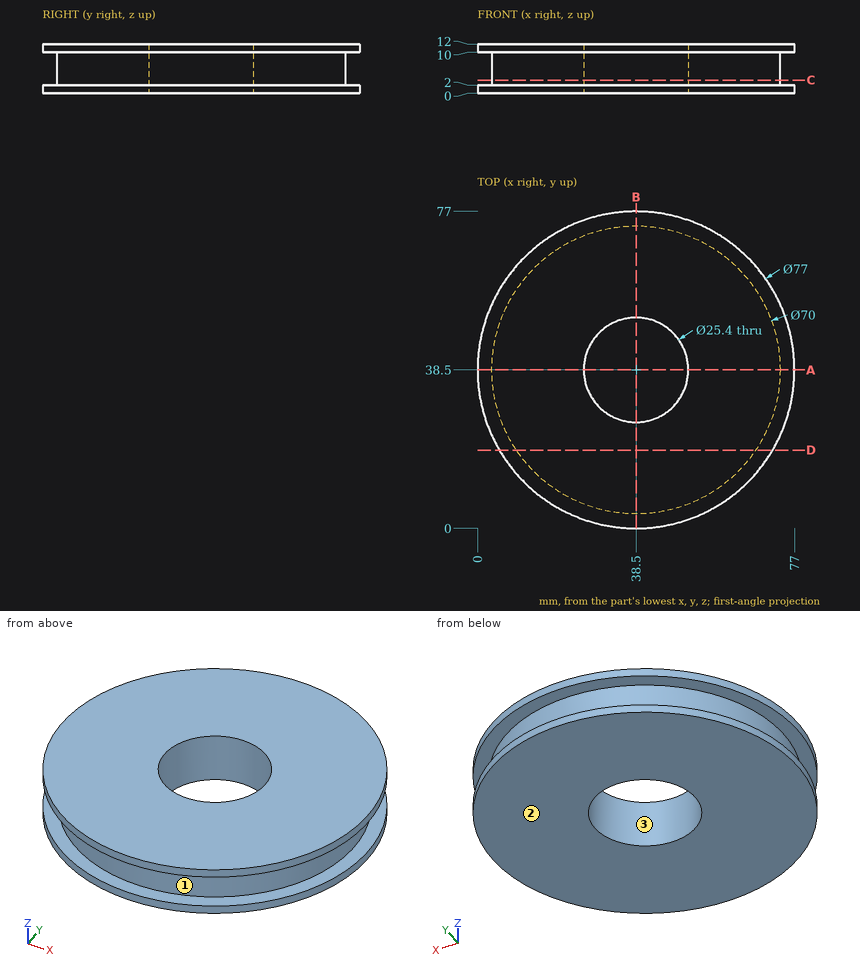
Geometry check sheet. Reference: drawing and pictorial views, mm from the part's lowest x, y, z. Round coordinates to 2 decimals unless told otherwise and drop trailing zeros. Loops run counter-clockwise (first coordinate to the right, second up) from the corner with the lowest first, then second, coordinate; pieces in that order, holes last. Notation, with made-up numbers: M -15,64 L 28,64 A10 cw 28,82 Z; hole C 71.5,66.5 d9. An arc over 180 degrees is marked long. Return JSON: item names as keys, results as strings. Group by question number.
(1) Go/stop test with flat-tipped pins: pin 1 (4 mm diameter, centred on x = 50, y = 24.5, fed in from -Z); pin 2 (1 mm diameter, centred on y = 22, z = 6.5, fed in from +X); pin 3 (6 mm diameter, centred on x = 34, z = 3, fed in from -Y); pin 4 (2 mm diameter, centred on y = 67, z = 2, fed in from -X). Record where each tip stops, or that it passes through.
(2) Section check A-A, the plane y = 38.5. Enter the section's corners in (x, z).
(3) Section check D-D, the plane y = 19. Enter the section's corners in (x, z).
(4) Scan lines: line 1 along Y through (x, z) = (38.5, 6.5); line 2 along Z through (x, y) = (74, 30); line 3 along Y through (x, z) = (50, 7). Record each from-to range of solid material in increasing order. Write a range as [from, to].
(5) Mould release check, pull along Y, two halves, no side actions. Record for the marked faces 1, 2 and 3: pulls with the +Y half, pulls with the -Y half, needs draft (parallel to the pull), parting line crosses it, or undercut.
(6) Section check C-C, the plane z = 3.25. Enter the section's corners in (x, y), and give its area (3 significant figures).
Data:
{
 "1": {"pin 1": "z = 0", "pin 2": "x = 69.63", "pin 3": "y = 0.04", "pin 4": "x = 11.56"},
 "2": {"outline": "M 0,0 L 25.8,0 L 25.8,12 L 0,12 L 0,10 L 3.5,10 L 3.5,2 L 0,2 Z; M 51.2,0 L 77,0 L 77,2 L 73.5,2 L 73.5,10 L 77,10 L 77,12 L 51.2,12 Z"},
 "3": {"outline": "M 5.3,0 L 71.7,0 L 71.7,2 L 67.56,2 L 67.56,10 L 71.7,10 L 71.7,12 L 5.3,12 L 5.3,10 L 9.44,10 L 9.44,2 L 5.3,2 Z"},
 "4": {"line 1": "[3.5, 25.8], [51.2, 73.5]", "line 2": "[0, 2], [10, 12]", "line 3": "[5.44, 33.11], [43.89, 71.56]"},
 "5": {"face 1": "parting line crosses it", "face 2": "needs draft", "face 3": "undercut"},
 "6": {"outline": "C 38.5,38.5 d70; hole C 38.5,38.5 d25.4", "area": "3,340 mm²"}
}
